Check sheet for the modelled part. Datum: model origin and axes. Units: mm. A direction names the side the tool comes from. Give positions to 0.01 mm unless a question says otherwise; leave off trailing zeros. Write each loop counter-clockwise with the first axis right and the second up, starting at its lowest first coordinate (ties: lowest second). Pieces come first, ordered by that corner, then holes. Notation, with made-up numbers: (71, 49) -> (93, 49) arc R38 ccw to (93, 88) -> close; hole circle Ø7 at (-33.75, 33.25). An arc over 180 degrees is marked (long way). Use a Markdown table: item, result. Add a question column.
1. Cross-section at B-B (x = 10.05). Enter the section's corners in (y, z), then the cut area to 3 significant figures.
2. Cross-section at D-D (x = 40). Enter the section's corners in (y, z).
3. Cross-section at A-A (x = -59.95). Enter the section's corners in (y, z).
4. Release check for a two-part mould opening along Y. For faces 1 (the cylindrical face through (66.55, 0.86, 2.46)), 2 (the cylindrical face through (6.235, 6.299, 4.26)), 3 (the flat face through (-1, 43, 5)), 4 (the cylindrical face through (-66.55, 84.04, 2.46)) record: released by +Y, released by -Y, zero draft, split by the parting line, or undercut.
5. Gauge pin test, flat end, axial feed: P1, Ø6.5, axis at x = -59.5, y = 7, coming from the +Z side. Record the tip position at first contact, or that the pin passes through.
6. Cross-section at C-C (y = 46.5). Enter the section's corners in (x, z), then the cut area to 4 significant figures.
7. Scan lines: probe 1 along X at (y, z) = (46.5, 3.35); probe 2 along X at (y, z) = (76.5, 3.8); probe 3 along Y at (x, z) = (59.95, 3.9). Record each from-to range of solid material in increasing order. Write a range as [from, to].
8. Set-up check for faces 5 (the flat face through (35.5, 43, 4)), 6 (the cylindrical face through (-63.765, 6.299, 4.26)), 7 (the flat face through (57.8, 78.1, 2)), 8 (the cylindrical face through (66.59, 84, 2.46)): record each of +Z, -Z, +X, -X, +Y, -Y from which the full face is reachable in a straight line by a thin tool's end or side.
from build123d import *

# Parameters (mm, degrees)
EXTRUDE_1_DEPTH     = 5
CUT_EXTRUDE_1_DEPTH = 2
SKETCH_3_R          = 2.05
CUT_EXTRUDE_2_DEPTH = 3
SKETCH_4_R          = 4
CUT_EXTRUDE_3_DEPTH = 1.5
SKETCH_5_W          = 6
SKETCH_5_H          = 10
CUT_EXTRUDE_4_DEPTH = 3
CUT_EXTRUDE_5_DEPTH = 3
CUT_EXTRUDE_START   = -3
CUT_EXTRUDE_6_DEPTH = 3


with BuildPart() as part:
    # 草图1 → 凸台-拉伸1 (new body)
    with BuildSketch(Plane.XY):
        with BuildLine():
            Line((-64.45, 0), (64.45, 0))
            ThreePointArc((64.45, 0), (66.571320344, 0.878679656), (67.45, 3))
            Line((67.45, 3), (67.45, 81.9))
            ThreePointArc((67.45, 81.9), (66.571320344, 84.021320344), (64.45, 84.9))
            Line((64.45, 84.9), (-64.45, 84.9))
            ThreePointArc((-64.45, 84.9), (-66.571320344, 84.021320344), (-67.45, 81.9))
            Line((-67.45, 81.9), (-67.45, 3))
            ThreePointArc((-67.45, 3), (-66.571320344, 0.878679656), (-64.45, 0))
        make_face()
    extrude(amount=EXTRUDE_1_DEPTH)

    # 草图2 → 切除-拉伸1 (cut)
    with BuildSketch(Plane(origin=(0, 0, 0), x_dir=(-1, 0, 0), z_dir=(0, 0, -1))):
        Polygon((-56.659103466, 77.4), (-58.304551733, 80.25), (-61.595448267, 80.25), (-63.240896534, 77.4), (-61.595448267, 74.55), (-58.304551733, 74.55), align=None)
        Polygon((58.304551733, 74.55), (56.659103466, 77.4), (58.304551733, 80.25), (61.595448267, 80.25), (63.240896534, 77.4), (61.595448267, 74.55), align=None)
        Polygon((-13.340896534, 7.5), (-11.695448267, 4.65), (-8.404551733, 4.65), (-6.759103466, 7.5), (-8.404551733, 10.35), (-11.695448267, 10.35), align=None)
        Polygon((56.659103466, 7.5), (58.304551733, 4.65), (61.595448267, 4.65), (63.240896534, 7.5), (61.595448267, 10.35), (58.304551733, 10.35), align=None)
    extrude(amount=-CUT_EXTRUDE_1_DEPTH, mode=Mode.SUBTRACT)

    # 草图3 → 切除-拉伸2 (cut)
    with BuildSketch(Plane(origin=(0, 0, 2), x_dir=(-1, 0, 0), z_dir=(0, 0, -1))):
        with Locations((-59.95, 77.4)):
            Circle(SKETCH_3_R)
        with Locations(Location((59.95, 77.4, 0), (0, 0, 180))):
            Circle(SKETCH_3_R)
        with Locations((-10.05, 7.5)):
            Circle(SKETCH_3_R)
        with Locations((59.95, 7.5)):
            Circle(SKETCH_3_R)
    extrude(amount=-CUT_EXTRUDE_2_DEPTH, mode=Mode.SUBTRACT)

    # 草图4 → 切除-拉伸3 (cut)
    with BuildSketch(Plane.XY.offset(5)):
        with Locations((-59.95, 77.4)):
            Circle(SKETCH_4_R)
        with Locations((59.95, 77.4)):
            Circle(SKETCH_4_R)
        with Locations(Location((-59.95, 7.5, 0), (0, 0, 180))):
            Circle(SKETCH_4_R)
        with Locations(Location((10.05, 7.5, 0), (0, 0, 180))):
            Circle(SKETCH_4_R)
    extrude(amount=-CUT_EXTRUDE_3_DEPTH, mode=Mode.SUBTRACT)

    # 草图5 → 切除-拉伸4 (cut)
    with BuildSketch(Plane.XY.offset(5)):
        with Locations((-41.5, 43)):
            Rectangle(SKETCH_5_W, SKETCH_5_H)
        with Locations((41.5, 43)):
            Rectangle(SKETCH_5_W, SKETCH_5_H)
    extrude(amount=-CUT_EXTRUDE_4_DEPTH, mode=Mode.SUBTRACT)

    # 草图6 → 切除-拉伸5 (cut)
    with BuildSketch(Plane(origin=(38.5, 0, 0), x_dir=(0, 0, -1), z_dir=(1, 0, 0))):
        with BuildLine():
            Line((-4.768857754, 43.8), (-5, 43.8))
            Line((-5, 43.8), (-5, 42.2))
            Line((-5, 42.2), (-4.768857754, 42.2))
            ThreePointArc((-4.768857754, 42.2), (-2, 43), (-4.768857754, 43.8))
        make_face()
    extrude(amount=-CUT_EXTRUDE_5_DEPTH, mode=Mode.SUBTRACT)

    # 草图7 → 切除-拉伸6 (cut)
    with BuildSketch(Plane.ZY.offset(38.5).offset(CUT_EXTRUDE_START)):
        with BuildLine():
            Line((5, 43.8), (4.768857754, 43.8))
            ThreePointArc((4.768857754, 43.8), (2, 43), (4.768857754, 42.2))
            Line((4.768857754, 42.2), (5, 42.2))
            Line((5, 42.2), (5, 43.8))
        make_face()
    extrude(amount=CUT_EXTRUDE_6_DEPTH, mode=Mode.SUBTRACT)


solid = part.part
Worked answers:
| question | item | result |
|---|---|---|
| 1 | outline | (0, 0) -> (4.65, 0) -> (4.65, 2) -> (5.45, 2) -> (5.45, 3.5) -> (3.5, 3.5) -> (3.5, 5) -> (0, 5) -> close; (9.55, 2) -> (10.35, 2) -> (10.35, 0) -> (84.9, 0) -> (84.9, 5) -> (11.5, 5) -> (11.5, 3.5) -> (9.55, 3.5) -> close |
| 1 | area | 395 mm² |
| 2 | outline | (0, 0) -> (84.9, 0) -> (84.9, 5) -> (48, 5) -> (48, 2) -> (38, 2) -> (38, 5) -> (0, 5) -> close |
| 3 | outline | (0, 0) -> (4.65, 0) -> (4.65, 2) -> (5.45, 2) -> (5.45, 3.5) -> (3.5, 3.5) -> (3.5, 5) -> (0, 5) -> close; (9.55, 2) -> (10.35, 2) -> (10.35, 0) -> (74.55, 0) -> (74.55, 2) -> (75.35, 2) -> (75.35, 3.5) -> (73.4, 3.5) -> (73.4, 5) -> (11.5, 5) -> (11.5, 3.5) -> (9.55, 3.5) -> close; (79.45, 2) -> (80.25, 2) -> (80.25, 0) -> (84.9, 0) -> (84.9, 5) -> (81.4, 5) -> (81.4, 3.5) -> (79.45, 3.5) -> close |
| 4 | face 1 | released by -Y |
| 4 | face 2 | undercut |
| 4 | face 3 | zero draft |
| 4 | face 4 | released by +Y |
| 5 | P1 | stops at z = 3.5 |
| 6 | outline | (-67.45, 0) -> (67.45, 0) -> (67.45, 5) -> (44.5, 5) -> (44.5, 2) -> (38.5, 2) -> (38.5, 5) -> (-38.5, 5) -> (-38.5, 2) -> (-44.5, 2) -> (-44.5, 5) -> (-67.45, 5) -> close |
| 6 | area | 638.5 mm² |
| 7 | probe 1 | x = [-67.45, -44.5], [-38.5, 38.5], [44.5, 67.45] |
| 7 | probe 2 | x = [-67.45, -63.85], [-56.05, 56.05], [63.85, 67.45] |
| 7 | probe 3 | y = [0, 73.4], [81.4, 84.9] |
| 8 | face 5 | none |
| 8 | face 6 | +Z |
| 8 | face 7 | -Z |
| 8 | face 8 | +Z, -Z, +X, +Y |
